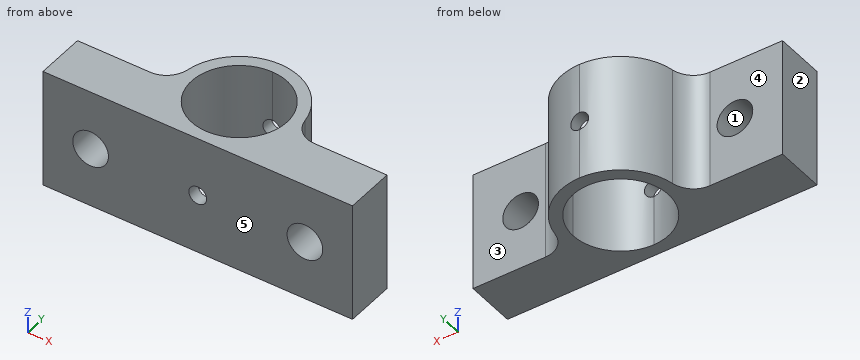
from build123d import *
from build123d.topology import SkipClean

# Parameters (mm, degrees)
BOSS_EXTRUDE1_DEPTH     = 10
SKETCH2_R               = 1.5
CUT_EXTRUDE1_DEPTH      = 10
CUT_EXTRUDE2_DEPTH      = 18.411616553
CUT_EXTRUDE2_DEPTH_BACK = 18.411616553
SKETCH3_R               = 0.75


with BuildPart() as part:
    # Sketch1 → Boss-Extrude1 (new body)
    with BuildSketch(Plane.XY):
        with BuildLine():
            Line((0, 1), (0, 0))
            Line((0, 0), (13, 0))
            Line((13, 0), (13, 4.154968692))
            Line((13, 4.154968692), (6.904060206, 4.154968692))
            ThreePointArc((6.904060206, 4.154968692), (5.611771946, 4.62853787), (4.931471575, 5.824977637))
            ThreePointArc((4.931471575, 5.824977637), (3.230720648, 8.816077055), (0, 10))
            Line((0, 10), (0, 9))
            ThreePointArc((0, 9), (2.828427125, 7.828427125), (4, 5))
            ThreePointArc((4, 5), (2.828427125, 2.171572875), (0, 1))
        make_face()
        with BuildLine():
            Line((-13, 0), (0, 0))
            Line((0, 0), (0, 1))
            ThreePointArc((0, 1), (-4, 5), (0, 9))
            Line((0, 9), (0, 10))
            ThreePointArc((0, 10), (-3.230720648, 8.816077055), (-4.931471575, 5.824977637))
            ThreePointArc((-4.931471575, 5.824977637), (-5.611771946, 4.62853787), (-6.904060206, 4.154968692))
            Line((-6.904060206, 4.154968692), (-13, 4.154968692))
            Line((-13, 4.154968692), (-13, 0))
        make_face()
    extrude(amount=BOSS_EXTRUDE1_DEPTH)

    # Sketch2 → Cut-Extrude1 (cut)
    with BuildSketch(Plane(origin=(0, 4.154968692, 0), x_dir=(1, 0, 0), z_dir=(0, 1, 0))):
        with Locations(Location((-9, -5, 0), (0, 0, 270))):
            Circle(SKETCH2_R)
        with Locations(Location((9, -5, 0), (0, 0, 270))):
            Circle(SKETCH2_R)
    extrude(amount=-CUT_EXTRUDE1_DEPTH, mode=Mode.SUBTRACT)

    # Sketch3 → Cut-Extrude2 (cut, two sides: drawn at the far end of the back side and taken through both)
    with SkipClean():  # the faces are left unmerged after this step: merging them gives an invalid solid
        with BuildSketch(Plane(origin=(0, 4.154968692, 0), x_dir=(1, 0, 0), z_dir=(0, 1, 0)).offset(-CUT_EXTRUDE2_DEPTH_BACK)):
            with Locations(Location((0, -5, 0), (0, 0, 270))):
                Circle(SKETCH3_R)
        extrude(amount=CUT_EXTRUDE2_DEPTH + CUT_EXTRUDE2_DEPTH_BACK, mode=Mode.SUBTRACT)


solid = part.part
Part model, mm, in its own coordinate system. Face numbers are marked on the shaded views. A direction names the side the tool comes from. Coordinates: 2 decimals unless noted, no trailing zeros. Loops run counter-clockwise (first coordinate to the right, second up) from the corner with the lowest first, then second, coordinate; pieces in that order, holes last. Notation, with made-up numbers: M 39.25,53.5 L 95.25,53.5 A24 cw 95.25,92.5 Z; hole C 38.25,47 d11. An arc over 180 degrees is marked long. Use a Markdown table: item, result. Add a question column.
Q1. Probe L1, parallel to X at y = 0.9, z = 5; L2, parallel to Z at x = 0, y = 0.6; L3, parallel to Y at x = -10.5, z = 2. List the from-to ranges inside material, lowest first.
Q2. Which spindle directions (+Z, -Z, +X, -X, +Y, -Y) get a long thin tool onto all of the face, cutting with end or side? Do the marked faces 4 and 5. Say none if no direction does.
Q3. Mould opens along X. For the marked faces 1, 2 and 3 say: +X half, -X half, draft (parallel to the pull), parting line (faces both ways), or undercut.
Q4. Cut at B-B (x = 9). Write the cut outline in (y, z).
Q5. Cut at D-D (z = 6). Write the cut outline in (x, y), and give its area (3 significant figures).
Q6. Pin check, flat tips, straight feed: P1, Ø3, axis at x = -6, y = 5, coming from the -Z side; P2, Ø1.2, axis at x = 0, z = 5, coming from the -Y side; P3, Ø3, axis at x = -9, z = 6, coming from the +Y side. Stop position of each tip, or through.
Q7. Cut at A-A (z = 8.5). Write the cut outline in (x, y), and give its area (3 significant figures).
Q8. Cut at C-C (y = 2.5). Write the cut outline in (x, z), and give its area (3 significant figures).
Worked out:
| question | item | result |
|---|---|---|
| 1 | L1 | x = -13 to -10.5, -7.5 to -0.75, 0.75 to 7.5, 10.5 to 13 |
| 1 | L2 | z = 0 to 4.25, 5.75 to 10 |
| 1 | L3 | y = 0 to 4.15 |
| 2 | face 4 | +Z, -Z, -X, +Y |
| 2 | face 5 | +Z, -Z, +X, -X, -Y |
| 3 | face 1 | undercut |
| 3 | face 2 | -X half |
| 3 | face 3 | draft |
| 4 | outline | M 0,0 L 4.15,0 L 4.15,3.5 L 0,3.5 Z; M 0,6.5 L 4.15,6.5 L 4.15,10 L 0,10 Z |
| 5 | outline | M -13,0 L -10.12,0 L -10.12,4.15 L -13,4.15 Z; M -7.88,0 L 7.88,0 L 7.88,4.15 L 6.9,4.15 A2 cw 4.93,5.82 A5 ccw -4.93,5.82 A2 cw -6.9,4.15 L -7.88,4.15 Z; M 10.12,0 L 13,0 L 13,4.15 L 10.12,4.15 Z; hole C 0,5 d8 |
| 5 | area | 88.3 mm2 |
| 6 | P1 | stops at z = 0 |
| 6 | P2 | passes through |
| 6 | P3 | stops at y = 4.15 |
| 7 | outline | M -13,0 L 13,0 L 13,4.15 L 6.9,4.15 A2 cw 4.93,5.82 A5 ccw -4.93,5.82 A2 cw -6.9,4.15 L -13,4.15 Z; hole C 0,5 d8 |
| 7 | area | 107 mm2 |
| 8 | outline | M -13,0 L -3.12,0 L -3.12,10 L -13,10 Z; M 3.12,0 L 13,0 L 13,10 L 3.12,10 Z; hole C -9,5 d3; hole C 9,5 d3 |
| 8 | area | 183 mm2 |
